CAD build for the part. Positions are in the model's coordinates, mm. Round coordinates to 2 decimals unless told otherwise and drop trailing zeros. Loops run counter-clockwise (first coordinate to the right, second up) from the corner with the lowest first, then second, coordinate; pieces in that order, holes last. Notation, with made-up numbers: (88, -9.5) - (143, -9.5) arc R19 ccw to (143, 24.5) - close; hole circle Ø10 at (24.5, 84.5). An arc over 180 degrees is marked (long way). Use one line per item in the form item = value.
from build123d import *

# Parameters (mm, degrees)
F0_W     = 82.204894
F0_H     = 67.080438
F1_DEPTH = 62.079741
F2_R     = 12.7
F3_R     = 12.7
F4_R     = 12.7


with BuildPart() as f1:
    # F0 (on Front) → F1 (new body)
    with BuildSketch(Plane.XZ):
        Rectangle(F0_W, F0_H)
    extrude(amount=F1_DEPTH)

    # F2
    f2_edges = [f1.edges().sort_by_distance(p)[0] for p in [
        (0, -62.079741, 33.540219),
    ]]
    fillet(f2_edges, radius=F2_R)

    # F3
    f3_edges = [f1.edges().sort_by_distance(p)[0] for p in [
        (0, -62.079741, -33.540219),
    ]]
    fillet(f3_edges, radius=F3_R)

    # F4
    f4_edges = [f1.edges().sort_by_distance(p)[0] for p in [
        (0, 0, -33.540219),
        (0, 0, 33.540219),
    ]]
    fillet(f4_edges, radius=F4_R)


solid = f1.part
1) Slice it at B-B (z = -27.5). Write the cut outline in (x, y), plus the area to 3 significant figures.
Report:
outline = (-41.1, -60.19) - (41.1, -60.19) - (41.1, -1.89) - (-41.1, -1.89) - close
area = 4,790 mm^2
2) Slice it at A-A (x = 16). Write the cut outline in (y, z), plus the area to 3 significant figures.
Report:
outline = (-62.08, -20.84) arc R12.7 ccw to (-49.38, -33.54) - (-12.7, -33.54) arc R12.7 ccw to (0, -20.84) - (0, 20.84) arc R12.7 ccw to (-12.7, 33.54) - (-49.38, 33.54) arc R12.7 ccw to (-62.08, 20.84) - close
area = 4,030 mm^2
3) Slice it at C-C (y = -8). Write the cut outline in (x, z), plus the area to 3 significant figures.
Report:
outline = (-41.1, -32.64) - (41.1, -32.64) - (41.1, 32.64) - (-41.1, 32.64) - close
area = 5,370 mm^2
4) Two-plate mould, pull along X, no slides. Class faces 1 (the flat face through (41.102, -31, 0)), 2 (the flat face through (-1, -31, 33.54)), 3 (the flat face through (-41.102, -31, 0)): +X half, -X half, draft (parallel to the pull), parting line (faces both ways), or undercut.
Report:
face_1 = +X half
face_2 = draft
face_3 = -X half
5) Drill centre lines: probe 1 along Z at (x, y) = (5, -50); probe 2 along Z at (x, y) = (-34, -6); probe 3 along Y at (x, z) = (-17, 25.5). Where is each one in solid material? Low to high.
Report:
probe_1 = -33.53 to 33.53
probe_2 = -31.63 to 31.63
probe_3 = -61.19 to -0.89
